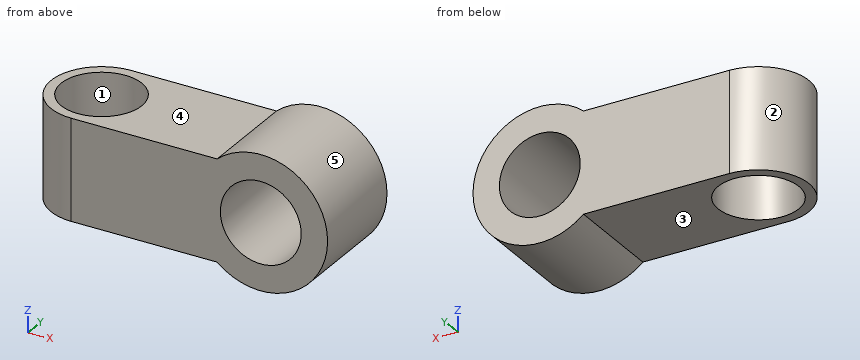
from build123d import *

# Parameters (mm, degrees)
SKETCH_1_R          = 3.305414419
SKETCH_1_R_2        = 2
EXTRUDE_1_DEPTH     = 5
EXTRUDE_2_DEPTH     = 2.5
CUT_EXTRUDE_START   = -5
SKETCH_5_R          = 2
CUT_EXTRUDE_1_DEPTH = 5
SKETCH_6_R          = 2
CUT_EXTRUDE_2_DEPTH = 15.112515325


with BuildPart() as part:
    # 草图1 → 凸台-拉伸1 (new body)
    with BuildSketch(Plane(origin=(0, 0, 0), x_dir=(1, 0, 0), z_dir=(0, 1, 0))):
        with Locations(Location((0, 0, 0), (0, 0, 270))):
            Circle(SKETCH_1_R)
        with Locations(Location((0, 0, 0), (0, 0, 270))):
            Circle(SKETCH_1_R_2, mode=Mode.SUBTRACT)
    extrude(amount=EXTRUDE_1_DEPTH)

    # 草图4 → 凸台-拉伸2 (add, symmetric)
    with BuildSketch(Plane.XY):
        with BuildLine():
            Line((0, 0), (0, 5))
            Line((0, 5), (-9.380296623, 5))
            ThreePointArc((-9.380296623, 5), (-11.851592814, 2.5), (-9.380296623, 0))
            Line((-9.380296623, 0), (0, 0))
        make_face()
    extrude(amount=EXTRUDE_2_DEPTH, both=True)

    # 草图5 → 切除-拉伸1 (cut)
    with BuildSketch(Plane(origin=(0, 5, 0), x_dir=(1, 0, 0), z_dir=(0, 1, 0)).offset(CUT_EXTRUDE_START)):
        with Locations(Location((0, 0, 0), (0, 0, 270))):
            Circle(SKETCH_5_R)
    extrude(amount=CUT_EXTRUDE_1_DEPTH, mode=Mode.SUBTRACT)

    # 草图6 → 切除-拉伸2 (cut, through all)
    with BuildSketch(Plane.XY.offset(2.5)):
        with Locations((-9.351426118, 2.5)):
            Circle(SKETCH_6_R)
    extrude(amount=-CUT_EXTRUDE_2_DEPTH, mode=Mode.SUBTRACT)


solid = part.part
The model under review builds one solid part; all positions refer to its coordinate system, in mm. Face numbers are marked on the shaded views. A direction names the side the tool comes from. Give positions to 0.01 mm unless a question says otherwise; leave off trailing zeros. Loops run counter-clockwise (first coordinate to the right, second up) from the corner with the lowest first, then second, coordinate; pieces in that order, holes last. Notation, with made-up numbers: (75.25, -17) -> (87.25, -17) arc R16 ccw to (87.25, -6) -> close; hole circle Ø8 at (2.5, 24). An arc over 180 degrees is marked (long way). Write each question's results on one line, items separated by ' | '.
1) For line 1 along X through (y, z) = (1.65, 0); line 2 along X through (y, z) = (3.2, -1.25); line 3 along Y through (x, z) = (-8, -1.5), list the stretches that pass through material, from the lowest coordinate up. Write a range as from..to.
Conclusion:
line 1: x = -11.7..-11.16, -7.54..-2, 2..3.31 | line 2: x = -11.75..-11.22, -7.48..-1.56, 1.56..3.06 | line 3: y = 0..1.03, 3.97..5
2) Take a section at B-B, the plane y = 2.5. Give the boundary of the cut face in (x, z).
Conclusion:
outline: (-11.85, -2.5) -> (-11.35, -2.5) -> (-11.35, 2.5) -> (-11.85, 2.5) -> close; (-7.35, -2.5) -> (-2.16, -2.5) arc R3.31 ccw (long way) to (-2.16, 2.5) -> (-7.35, 2.5) -> close; hole circle Ø4 at (0, 0)
3) Tool access review of the marked faces 4 and 5: name each direction out of +Z, -Z, +X, -X, +Y, -Y from which nothing blocks a thin tool from reaching the whole face with its end or side.
Conclusion:
face 4: +Z, -X, +Y, -Y | face 5: +Y, -Y
4) Draft analysis for pull direction X (two halves, no side actions). For the marked faces 1, 2 and 3, state which applies: pulls with the +X half, pulls with the -X half, needs draft (parallel to the pull), parting line crosses it, or undercut.
Conclusion:
face 1: undercut | face 2: pulls with the -X half | face 3: needs draft
5) Take a section at A-A, the plane z = 0. Give the boundary of the cut face in (x, y).
Conclusion:
outline: (-9.38, 0) -> (-2, 0) -> (-2, 5) -> (-9.38, 5) arc R2.5 ccw to start; (2, 0) -> (3.31, 0) -> (3.31, 5) -> (2, 5) -> close; hole circle Ø4 at (-9.35, 2.5)
6) Take a section at D-D, the plane x = -4. Give the boundary of the cut face in (y, z), plus the area to 3 significant figures.
Conclusion:
outline: (0, -2.5) -> (5, -2.5) -> (5, 2.5) -> (0, 2.5) -> close | area: 25.0 mm^2
7) Take a section at C-C, the plane x = 0. Give the boundary of the cut face in (y, z), plus the area to 3 significant figures.
Conclusion:
outline: (0, -3.31) -> (5, -3.31) -> (5, -2) -> (0, -2) -> close; (0, 2) -> (5, 2) -> (5, 3.31) -> (0, 3.31) -> close | area: 13.1 mm^2
8) Insertion check: pin 1 Ø3 at (x, y) = (-9.35, 2.5) entering from -Z; pin 2 Ø2.5 at (x, y) = (-7, 1.5) entering from -Z. Each pin has a flat end and moves straight along its axis. Give the tip position at first contact, or say it passes through.
Conclusion:
pin 1: passes through | pin 2: stops at z = -2.5
